from build123d import *

# Parameters (mm, degrees)
F0_W     = 19.05
F0_H     = 19.05
F0_R     = 6.35
F1_DEPTH = 25.4


with BuildPart() as f1:
    # F0 (on Front) → F1 (new body)
    with BuildSketch(Plane.XZ):
        with Locations((-15.875, -15.875)):
            Rectangle(F0_W, F0_H)
        Polygon((-6.35, -6.35), (-6.35, -25.4), (25.4, -25.4), (25.4, 25.4), (-25.4, 25.4), (-25.4, -6.35), align=None)
        Circle(F0_R, mode=Mode.SUBTRACT)
        Polygon((0, 53.798063), (-25.4, 25.4), (25.4, 25.4), align=None)
    extrude(amount=F1_DEPTH)


solid = f1.part
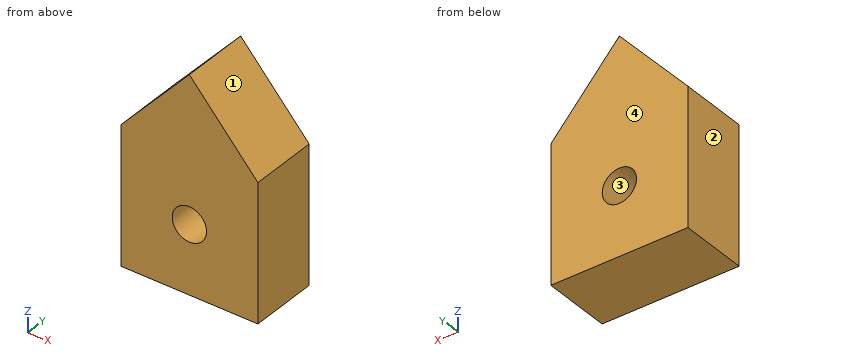
Model file for the job. Use its own axes, mm. Face numbers are marked on the shaded views. Round coordinates to 2 decimals unless told otherwise and drop trailing zeros. Order: outer loops, then holes, each group sorted by start corner. A loop starts at its lowest first (then second) coordinate and runs counter-clockwise, first axis right, second up. Notation, with made-up numbers: M 14.5,-20 L 19.5,-20 A32 ccw 19.5,16 Z; hole C 69.5,17 d9. An arc over 180 degrees is marked long. Write each question's results on one line, items separated by ' | '. Start each with the question number.
(1) Saw through at C-C, the plane x = 1. Give the cut face in (y, z), then the cut area to 3 significant figures.
(2) Saw through at B-B, the plane y = -16.75. Give the cut face in (x, z).
(3) Probe probe 1 along Z at (x, y) = (0, -13.25); probe 2 along X at (y, z) = (-17.25, 2); probe 3 along X at (y, z) = (-20.5, 4). List the from-to ranges inside material, lowest first. Write a range as from..to.
(4) Saw through at D-D, the plane x = 11.5. Give the cut face in (y, z), then the cut area to 3 significant figures.
(5) Two-plate mould, pull along X, no slides. Class the marked faces 1, 2, 3 and 4: pulls with the +X half, pulls with the -X half, needs draft (parallel to the pull), parting line crosses it, or undercut.
(6) Drop a flat-ended pin along its axis: pin 1 (3 mm diameter, centred on x = 7.5, z = -15.5, fed in from +Y). Give the stop position or say it passes through.
(7) Saw through at A-A, the plane z = 0. Give the cut face in (x, y), then the cut area to 3 significant figures.
Established:
1) outline: M -25.4,-25.4 L 0,-25.4 L 0,-6.27 L -25.4,-6.27 Z; M -25.4,6.27 L 0,6.27 L 0,52.68 L -25.4,52.68 Z | area: 1,660 mm^2
2) outline: M -25.4,-25.4 L 25.4,-25.4 L 25.4,25.4 L 0,53.8 L -25.4,25.4 Z; hole C 0,0 d12.7
3) probe 1: z = -25.4..-6.35, 6.35..53.8 | probe 2: x = -25.4..-6.03, 6.03..25.4 | probe 3: x = -25.4..-4.93, 4.93..25.4
4) outline: M -25.4,-25.4 L 0,-25.4 L 0,40.94 L -25.4,40.94 Z | area: 1,690 mm^2
5) face 1: pulls with the +X half | face 2: pulls with the -X half | face 3: undercut | face 4: needs draft
6) pin 1: stops at y = 0
7) outline: M -25.4,-25.4 L -6.35,-25.4 L -6.35,0 L -25.4,0 Z; M 6.35,-25.4 L 25.4,-25.4 L 25.4,0 L 6.35,0 Z | area: 968 mm^2
